Geometry: final body of the model. Coordinates: model frame, mm. A direction names the side the tool comes from. Give positions to 0.01 mm unless a question says otherwise; leave off trailing zeros. Write each loop counter-clockwise with the first axis right and the second up, starting at its lowest first coordinate (ties: lowest second). Pieces come first, ordered by that corner, then holes. Notation, with made-up numbers: (-38, -14.5) -> (-9, -14.5) arc R34 ccw to (-9, 18.5) -> close; hole circle Ø6 at (75.25, 47.5). An arc over 180 degrees is marked (long way). Answer as a JSON object with one key per item and string values.
from build123d import *

# Parameters (mm, degrees)
SKETCH1_W           = 33
SKETCH1_H           = 44
BOSS_EXTRUDE1_DEPTH = 21
SHELL1_START        = 2
SHELL1_OUTLINE_W    = 17
SHELL1_OUTLINE_H    = 40
SHELL1_DEPTH        = 29
SKETCH2_W           = 29.062005015
SKETCH2_H           = 39.767253615
CUT_EXTRUDE1_DEPTH  = 7
CUT_EXTRUDE2_DEPTH  = 7
SKETCH4_W           = 15
SKETCH4_H           = 3.175
CUT_EXTRUDE3_DEPTH  = 45
CHAMFER1_SIZE       = 2


# Read off the part's stored shape, not the designer's step: Shell1
with BuildPart() as part:
    # Sketch1 → Boss-Extrude1 (new body)
    with BuildSketch(Plane(origin=(0, 0, 0), x_dir=(1, 0, 0), z_dir=(0, 1, 0))):
        with Locations((16.5, -12.899591929)):
            Rectangle(SKETCH1_W, SKETCH1_H)
    extrude(amount=BOSS_EXTRUDE1_DEPTH)

    # Shell1 outline → Shell1 (cut)
    with BuildSketch(Plane.YZ.offset(SHELL1_START)):
        with Locations((10.5, 12.899591929)):
            Rectangle(SHELL1_OUTLINE_W, SHELL1_OUTLINE_H)
    extrude(amount=SHELL1_DEPTH, mode=Mode.SUBTRACT)

    # Sketch2 → Cut-Extrude1 (cut)
    with BuildSketch(Plane(origin=(0, 21, 0), x_dir=(1, 0, 0), z_dir=(0, 1, 0))):
        with Locations((16.531002507, -12.783218737)):
            Rectangle(SKETCH2_W, SKETCH2_H)
    extrude(amount=-CUT_EXTRUDE1_DEPTH, mode=Mode.SUBTRACT)

    # Sketch3 → Cut-Extrude2 (cut)
    with BuildSketch(Plane.XY.offset(34.899591929)):
        with BuildLine():
            ThreePointArc((14.5, 8.681065769), (12.889087297, 12.570153065), (9, 14.181065769))
            Line((9, 14.181065769), (9, 3.181065769))
            ThreePointArc((9, 3.181065769), (12.889087297, 4.791978472), (14.5, 8.681065769))
        make_face()
        with BuildLine():
            Line((9, 3.181065769), (9, 14.181065769))
            ThreePointArc((9, 14.181065769), (3.5, 8.681065769), (9, 3.181065769))
        make_face()
        with BuildLine():
            Line((16.5, 3.181065769), (16.5, 14.181065769))
            Line((16.5, 14.181065769), (9, 14.181065769))
            ThreePointArc((9, 14.181065769), (12.889087297, 12.570153065), (14.5, 8.681065769))
            ThreePointArc((14.5, 8.681065769), (12.889087297, 4.791978472), (9, 3.181065769))
            Line((9, 3.181065769), (16.5, 3.181065769))
        make_face()
        with BuildLine():
            ThreePointArc((24, 3.181065769), (18.5, 8.681065769), (24, 14.181065769))
            Line((24, 14.181065769), (16.5, 14.181065769))
            Line((16.5, 14.181065769), (16.5, 3.181065769))
            Line((16.5, 3.181065769), (24, 3.181065769))
        make_face()
        with BuildLine():
            ThreePointArc((29.5, 8.681065769), (27.889087297, 12.570153065), (24, 14.181065769))
            Line((24, 14.181065769), (24, 3.181065769))
            ThreePointArc((24, 3.181065769), (27.889087297, 4.791978472), (29.5, 8.681065769))
        make_face()
        with BuildLine():
            Line((24, 3.181065769), (24, 14.181065769))
            ThreePointArc((24, 14.181065769), (18.5, 8.681065769), (24, 3.181065769))
        make_face()
    extrude(amount=-CUT_EXTRUDE2_DEPTH, mode=Mode.SUBTRACT)

    # Sketch4 → Cut-Extrude3 (cut)
    with BuildSketch(Plane(origin=(33, 0, 0), x_dir=(0, 0, -1), z_dir=(1, 0, 0))):
        with Locations((-12.899591929, 19.4125)):
            Rectangle(SKETCH4_W, SKETCH4_H)
    extrude(amount=-CUT_EXTRUDE3_DEPTH, mode=Mode.SUBTRACT)

    # Chamfer1
    chamfer1_edges = [part.edges().sort_by_distance(p)[0] for p in [
        (16.5, 0, 34.899591929),
        (33, 0, 12.899591929),
        (16.5, 0, -9.100408071),
        (0, 0, 12.899591929),
        (33, 21, -1.850408071),
        (16.5, 21, -9.100408071),
        (0, 21, -1.850408071),
        (0, 21, 27.649591929),
        (16.5, 21, 34.899591929),
        (33, 21, 27.649591929),
    ]]
    chamfer(chamfer1_edges, length=CHAMFER1_SIZE - 0.0001)  # a hair under: the kernel refuses the full size


solid = part.part
Q1. Set-up query: faces 1 (the flat face through (16, 3.181, 34)), 2 (the flat face through (1, 19, 20.4)), 3 (the flat face through (16.3, 1, 33.9)). Return all of +Z, -Z, +X, -X, +Y, -Y with unobstructed straight access to the full face (end or side cutting, diameter ignored); none if empty.
Values:
{"face 1": "+Z", "face 2": "+X, -X, +Y", "face 3": "+Z, +X, -X, -Y"}
Q2. First-contact query: P1, Ø3, axis at x = 24, z = 5.5, coming from the +Y side; P2, Ø1, axis at x = 13.5, z = 33.5, coming from the +Y side; P3, Ø1, axis at x = 0.5, z = 15.5, coming from the +Y side (3 decimals). Flat tips, straight axial feed; report the tip coordinate or a pass-through.
Values:
{"P1": "y = 2", "P2": "y = 20.9", "P3": "y = 17.825"}
Q3. Material intervals for L1, parallel to Z at x = 12.5, y = 18; L2, parallel to X at y = 13.5, z = 28.5; L3, parallel to X at y = 18.25, z = 29, sorted ascending. Write a range as from..to.
Values:
{"L1": "-9.1..-7.1, 32.9..34.9", "L2": "0..2, 31..33", "L3": "0..2, 31.06..33"}
Q4. Cut plane A-A (y = 15). Return the cut outline in (x, z).
Values:
{"outline": "(0, -9.1) -> (33, -9.1) -> (33, 34.9) -> (0, 34.9) -> close; hole (2, -7.1) -> (31.06, -7.1) -> (31.06, 32.67) -> (31, 32.67) -> (31, 32.9) -> (2, 32.9) -> close"}
Q5. Mould query, pull axis Z, two halves, no side actions, for faces 4 (the flat face through (16, 20, 32.667)), 5 (the flat face through (16, 12, -7.1)), 6 (the flat face through (0, 10, 13)), 7 (the flat face through (16, 10, -9.1)). Classes: pulls with the +Z half, pulls with the -Z half, needs draft (parallel to the pull), parting line crosses it, or undercut.
Values:
{"face 4": "undercut", "face 5": "undercut", "face 6": "needs draft", "face 7": "pulls with the -Z half"}
